Part model, mm, in its own coordinate system. Face numbers are marked on the shaded views. A direction names the side the tool comes from. Give positions to 0.01 mm unless a question says otherwise; leave off trailing zeros. Write each loop counter-clockwise with the first axis right and the second up, starting at its lowest first coordinate (ties: lowest second). Pieces come first, ordered by that corner, then holes.
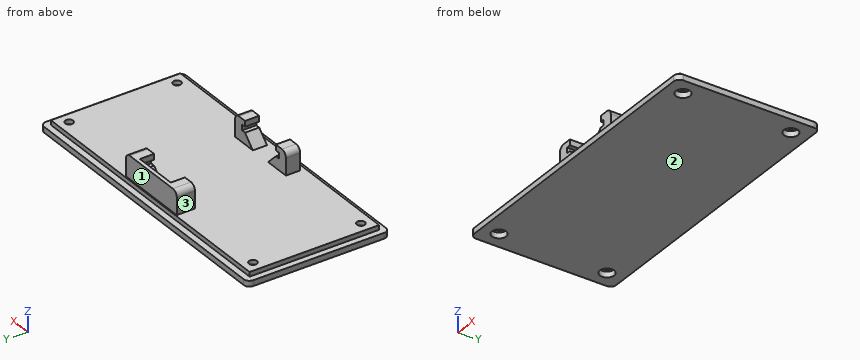
```python
from build123d import *

# Parameters (mm, degrees)
SKETCH_1_W                     = 106
SKETCH_1_H                     = 50
BODY_DEPTH                     = 2
SKETCH_2_W                     = 101.6
SKETCH_2_H                     = 45.6
INTERNALBODY_DEPTH             = 1.6
SKETCH_3_R                     = 1.4
HOLESCREW_DEPTH                = 59.710816721
SKETCH_3_3_R                   = 2.5
SKETCH_3_3_R_2                 = 1.4
TOPSCREWPLACE_DEPTH            = 2
SCREWMIRROR2_COPY_1_SKETCH_R   = 1.4
SCREWMIRROR2_COPY_1_DEPTH      = 59.710816721
SCREWMIRROR2_COPY_2_SKETCH_R   = 2.5
SCREWMIRROR2_COPY_2_SKETCH_R_2 = 1.4
SCREWMIRROR2_COPY_2_DEPTH      = 2
CORNERS_R                      = 2
SKETCH_4_W                     = 26
SKETCH_4_H                     = 1.4
ARDUINONANOSTOPS_DEPTH         = 8
ARDUINONANOHOLDER1_DEPTH       = 5
PATTERN_LINEAR_1_COUNT         = 2
PATTERN_LINEAR_1_PITCH         = 37
CHAMFER_1_SIZE                 = 4
FILLET_1_R                     = 2


with BuildPart() as part:
    # Эскиз1 → Body (new body)
    with BuildSketch(Plane.XY):
        Rectangle(SKETCH_1_W, SKETCH_1_H)
    extrude(amount=BODY_DEPTH)

    # Эскиз2 → InternalBody (add)
    with BuildSketch(Plane.XY.offset(2)):
        Rectangle(SKETCH_2_W, SKETCH_2_H)
    extrude(amount=INTERNALBODY_DEPTH)

    # Эскиз3 → HoleScrew (cut, through all)
    with BuildSketch(Plane(origin=(0, 0, 0), x_dir=(-1, 0, 0), z_dir=(0, 0, -1))):
        with Locations((47, -19)):
            Circle(SKETCH_3_R)
    holescrew = extrude(amount=-HOLESCREW_DEPTH, mode=Mode.SUBTRACT)

    # Эскиз3<3> → TopScrewPlace (cut)
    with BuildSketch(Plane(origin=(0, 0, 0), x_dir=(-1, 0, 0), z_dir=(0, 0, -1))):
        with Locations((47, -19)):
            Circle(SKETCH_3_3_R)
        with Locations((47, -19)):
            Circle(SKETCH_3_3_R_2, mode=Mode.SUBTRACT)
    topscrewplace = extrude(amount=-TOPSCREWPLACE_DEPTH, mode=Mode.SUBTRACT)

    # ScrewMrror1: HoleScrew, TopScrewPlace across plane
    add(holescrew.mirror(Plane.ZX), mode=Mode.SUBTRACT)
    add(topscrewplace.mirror(Plane.ZX), mode=Mode.SUBTRACT)

    # ScrewMirror2: HoleScrew, TopScrewPlace across plane
    add(holescrew.mirror(Plane(origin=(0, 0, 0), x_dir=(0, 0, 1), z_dir=(1, 0, 0))), mode=Mode.SUBTRACT)
    add(topscrewplace.mirror(Plane(origin=(0, 0, 0), x_dir=(0, 0, 1), z_dir=(1, 0, 0))), mode=Mode.SUBTRACT)

    # ScrewMirror2 copy 1 sketch → ScrewMirror2 copy 1 (cut, through all)
    with BuildSketch(Plane(origin=(0, 0, 0), x_dir=(1, 0, 0), z_dir=(0, 0, -1))):
        with Locations((47, -19)):
            Circle(SCREWMIRROR2_COPY_1_SKETCH_R)
    extrude(amount=-SCREWMIRROR2_COPY_1_DEPTH, mode=Mode.SUBTRACT)

    # ScrewMirror2 copy 2 sketch → ScrewMirror2 copy 2 (cut)
    with BuildSketch(Plane(origin=(0, 0, 0), x_dir=(1, 0, 0), z_dir=(0, 0, -1))):
        with Locations((47, -19)):
            Circle(SCREWMIRROR2_COPY_2_SKETCH_R)
        with Locations((47, -19)):
            Circle(SCREWMIRROR2_COPY_2_SKETCH_R_2, mode=Mode.SUBTRACT)
    extrude(amount=-SCREWMIRROR2_COPY_2_DEPTH, mode=Mode.SUBTRACT)

    # Corners
    corners_edges = [part.edges().sort_by_distance(p)[0] for p in [
        (53, -25, 1),
        (-53, -25, 1),
        (-53, 25, 1),
        (53, 25, 1),
    ]]
    fillet(corners_edges, radius=CORNERS_R)

    # Эскиз4 → ArduinoNanoStops (add)
    with BuildSketch(Plane.XY.offset(3.6)):
        with Locations((0, 21.7)):
            Rectangle(SKETCH_4_W, SKETCH_4_H)
    extrude(amount=ARDUINONANOSTOPS_DEPTH)

    # Эскиз5 → ArduinoNanoHolder1 (add)
    with BuildSketch(Plane.XZ.offset(-21)):
        Polygon((-7.9, 11.6), (-7.9, 9.6), (-9.4, 9.6), (-9.4, 7.6), (-7.9, 7.6), (-7.9, 3.6), (-13, 3.6), (-13, 11.6), align=None)
        Polygon((7.9, 11.6), (7.9, 9.6), (9.4, 9.6), (9.4, 7.6), (7.9, 7.6), (7.9, 3.6), (13, 3.6), (13, 11.6), align=None)
    arduinonanoholder1 = extrude(amount=ARDUINONANOHOLDER1_DEPTH)

    # Линейный массив1: ArduinoNanoHolder1 ×2
    with Locations(*[(0, -i * PATTERN_LINEAR_1_PITCH, 0) for i in range(1, PATTERN_LINEAR_1_COUNT)]):
        add(arduinonanoholder1)

    # Фаска1
    chamfer_1_edges = [part.edges().sort_by_distance(p)[0] for p in [
        (7.9, 18.5, 3.6),
        (7.9, -18.5, 3.6),
        (-7.9, -18.5, 3.6),
        (-7.9, 18.5, 3.6),
    ]]
    chamfer(chamfer_1_edges, length=CHAMFER_1_SIZE - 0.0001)  # a hair under: the kernel refuses the full size

    # Скругление1
    fillet_1_edges = [part.edges().sort_by_distance(p)[0] for p in [
        (-13, 19.2, 11.6),
        (13, 19.2, 11.6),
        (-13, -18.5, 11.6),
        (13, -18.5, 11.6),
    ]]
    fillet(fillet_1_edges, radius=FILLET_1_R)


solid = part.part
```
1) Pin check, flat tips, straight feed: pin 1 Ø1 at (y, z) = (-18, 10) entering from -X; pin 2 Ø6 at (x, y) = (-47, -19) entering from +Z; pin 3 Ø4 at (x, z) = (-20.5, 6.5) entering from -Y; pin 4 Ø0.6 at (y, z) = (-19, 9) entering from +X. Stop position of each tip, or through.
Answers follow:
pin 1: stops at x = -13
pin 2: stops at z = 3.6
pin 3: passes through
pin 4: stops at x = 13
2) 3-axis set-ups, long thin cutter, end or side, ignore diameter. For the marked faces 1, 2 and 3: which of +Z, -Z, +X, -X, +Y, -Y reach the whole face in a straight line?
Answers follow:
face 1: +Z, +X, -X, +Y
face 2: -Z, +X, -X, +Y, -Y
face 3: +Z, -X, +Y, -Y
3) Saw through at D-D, the plane y = -19. Count the separate pieces of the cut face and the enclosed holes in it, then the cut area to 3 significant figures.
Answers follow:
separate pieces: 3
enclosed holes: 0
area: 435 mm2
4) Saw through at C-C, the plane z = 5. Write the cut outline in (x, y).
Answers follow:
outline: (-13, -21) - (-5.3, -21) - (-5.3, -16) - (-13, -16) - close; (-13, 16) - (-5.3, 16) - (-5.3, 21) - (5.3, 21) - (5.3, 16) - (13, 16) - (13, 22.4) - (-13, 22.4) - close; (5.3, -21) - (13, -21) - (13, -16) - (5.3, -16) - close
5) Saw through at A-A, the plane x = -47. Write the cut outline in (y, z).
Answers follow:
outline: (-25, 0) - (-21.5, 0) - (-21.5, 2) - (-20.4, 2) - (-20.4, 3.6) - (-22.8, 3.6) - (-22.8, 2) - (-25, 2) - close; (-17.6, 2) - (-16.5, 2) - (-16.5, 0) - (16.5, 0) - (16.5, 2) - (17.6, 2) - (17.6, 3.6) - (-17.6, 3.6) - close; (20.4, 2) - (21.5, 2) - (21.5, 0) - (25, 0) - (25, 2) - (22.8, 2) - (22.8, 3.6) - (20.4, 3.6) - close
6) Wall check: L1, parallel to X at y = 19, z = 0.9; L2, parallel to X at y = 19, z = 3.1; L3, parallel to Y at x = -47, z = 2.8. Give the ranges that are in metal, low to high.
Answers follow:
L1: x = -53 to -49.5, -44.5 to 44.5, 49.5 to 53
L2: x = -50.8 to -48.4, -45.6 to 45.6, 48.4 to 50.8
L3: y = -22.8 to -20.4, -17.6 to 17.6, 20.4 to 22.8
7) Saw through at B-B, the plane y = 5. Write the cut outline in (x, z).
Answers follow:
outline: (-53, 0) - (53, 0) - (53, 2) - (50.8, 2) - (50.8, 3.6) - (-50.8, 3.6) - (-50.8, 2) - (-53, 2) - close
